from build123d import *

# Parameters (mm, degrees)
SKETCH2_R           = 15
BOSS_EXTRUDE1_DEPTH = 7.5


with BuildPart() as part:
    # Sketch2 → Boss-Extrude1 (new body, symmetric)
    with BuildSketch(Plane.XY):
        with BuildLine():
            Line((0, 0), (164, 0))
            Line((164, 0), (714, 116.906108919))
            Line((714, 116.906108919), (864, 116.906108919))
            ThreePointArc((864, 116.906108919), (919.084102522, 74.560174885), (892.323020072, 10.440903632))
            Line((892.323020072, 10.440903632), (727.653990867, -83.846064196))
            Line((727.653990867, -83.846064196), (571.872200418, -225.540335787))
            ThreePointArc((571.872200418, -225.540335787), (556.597798177, -232.94262163), (539.751135216, -230.87111334))
            Line((539.751135216, -230.87111334), (413.142119809, -175.969772575))
            ThreePointArc((413.142119809, -175.969772575), (376.982520463, -166.120087872), (339.620193825, -163.189309492))
            Line((339.620193825, -163.189309492), (249.620193825, -164.588795558))
            Line((249.620193825, -164.588795558), (249.620193825, -148.658795558))
            Line((249.620193825, -148.658795558), (225, -153))
            Line((225, -153), (0, -153))
            Line((0, -153), (0, 0))
        make_face()
        with Locations((551.686209295, -186.833379926)):
            Circle(SKETCH2_R, mode=Mode.SUBTRACT)
    extrude(amount=BOSS_EXTRUDE1_DEPTH, both=True)


solid = part.part
Can you work these out from the model? Positions are in its coordinate system, mm. A direction names the side the tool comes from. Round coordinates to 2 decimals unless told otherwise and drop trailing zeros. Write each loop counter-clockwise with the first axis right and the second up, starting at its lowest first coordinate (ties: lowest second). Pieces come first, ordered by that corner, then holes. Notation, with made-up numbers: M 63.25,89.5 L 72.25,89.5 A16 cw 72.25,110.5 Z; hole C 45.5,-18.5 d5. An arc over 180 degrees is marked long. Use CSV: the item, a comma, the result in double quotes.
(1) Imagine slicing it at A-A (z = -2.5). Write out the boundary of the cut face in (x, y), plus the area to 3 significant figures.
Check values:
outline,"M 0,-153 L 225,-153 L 249.62,-148.66 L 249.62,-164.59 L 339.62,-163.19 A200 cw 413.14,-175.97 L 539.75,-230.87 A30 ccw 571.87,-225.54 L 727.65,-83.85 L 892.32,10.44 A57 ccw 864,116.91 L 714,116.91 L 164,0 L 0,0 Z; hole C 551.69,-186.83 d30"
area,"183,000 mm^2"
(2) I'm going to push flat-ended pins straight in: pin 1 (4.5 mm diameter, centred on y = -154.5, z = -2.5, fed in from -X); pin 2 (4.5 mm diameter, centred on x = 137.5, z = 1.5, fed in from -Y); pin 3 (1 mm diameter, centred on y = 54.5, z = -5.5, fed in from +X); pin 4 (1 mm diameter, centred on y = -104.5, z = -4, fed in from +X). Where does each tip first touch, or does it pass through?
Check values:
pin 1,"x = 0"
pin 2,"y = -153"
pin 3,"x = 920.79"
pin 4,"x = 705.5"
(3) Imagine slicing it at C-C (y = -18). Write out the boundary of the cut face in (x, z), plus the area to 3 significant figures.
Check values:
outline,"M 0,-7.5 L 842.65,-7.5 L 842.65,7.5 L 0,7.5 Z"
area,"12,600 mm^2"
(4) Imagine slicing it at B-B (x = 91.5). Write out the boundary of the cut face in (y, z), plus the area to 4 significant figures.
Check values:
outline,"M -153,-7.5 L 0,-7.5 L 0,7.5 L -153,7.5 Z"
area,"2,295 mm^2"
(5) We'd pull the mould along X, two halves only. Please class faces 4 (the flat face through (237.48, -150.8, 0.11)), 5 (the cylindrical face through (918.806, 75.569, 0.105)), 6 (the flat face through (114, -153, 0)), 7 (the flat face through (477.333, -203.805, 0.105)): +X half, -X half, draft (parallel to the pull), parting line (faces both ways), or undercut.
Check values:
face 4,"undercut"
face 5,"+X half"
face 6,"draft"
face 7,"-X half"
(6) I need wall thicknesses on line 1 along Y through (x, z) = (90, 3.5); line 2 along Y through (x, z) = (200, -6.5); line 3 along X through (y, z) = (-113, -3.25). Which ranges of each line are inside material? Lowest first, please.
Check values:
line 1,"-153 to 0"
line 2,"-153 to 7.65"
line 3,"0 to 695.6"
(7) On a 3-axis mill with a long thin cutter (end or side, diameter ignored), from which of +Z, -Z, +X, -X, +Y, -Y can I reach the whole of each face in a straight line? I mean faces 1 (the cylindrical face through (377.5, -166.21, 0.11)), 2 (the flat face through (467, -56, 7.5)), 3 (the flat face through (81, 0, 0)). Say none if no direction works.
Check values:
face 1,"+Z, -Z, -Y"
face 2,"+Z, +X, -X, +Y, -Y"
face 3,"+Z, -Z, -X, +Y"
